Check sheet for the modelled part. Datum: model origin and axes. Units: mm. A direction names the side the tool comes from. Round coordinates to 2 decimals unless told otherwise and drop trailing zeros. Order: outer loops, then holes, each group sorted by start corner. A loop starts at its lowest first (then second) coordinate and runs counter-clockwise, first axis right, second up.
```python
from build123d import *

# Parameters (mm, degrees)
SKETCH3_R           = 2.225
BOSS_EXTRUDE1_DEPTH = 1.6


with BuildPart() as part:
    # Sketch1 → Revolve1 (revolve)
    with BuildSketch(Plane(origin=(0, 0, 0), x_dir=(1, 0, 0), z_dir=(0, 1, 0)), mode=Mode.PRIVATE) as revolve1_sk:
        with BuildLine():
            Line((0, -8.4), (0, 8.4))
            Line((0, 8.4), (1.725, 8.4))
            ThreePointArc((1.725, 8.4), (2.078553391, 8.253553391), (2.225, 7.9))
            Line((2.225, 7.9), (2.225, -7.9))
            ThreePointArc((2.225, -7.9), (2.078553391, -8.253553391), (1.725, -8.4))
            Line((1.725, -8.4), (0, -8.4))
        make_face()
    revolve(revolve1_sk.sketch.rotate(Axis((0, 0, -9.24), (0, 0, 1)), 180), axis=Axis((0, 0, -9.24), (0, 0, 1)))



with BuildPart() as body_2:
    # Sketch2 → Revolve2 (revolve)
    with BuildSketch(Plane.XZ, mode=Mode.PRIVATE) as revolve2_sk:
        with BuildLine():
            Line((-12.7, 8.4), (-14.425, 8.4))
            ThreePointArc((-14.425, 8.4), (-14.778553391, 8.253553391), (-14.925, 7.9))
            Line((-14.925, 7.9), (-14.925, -7.9))
            ThreePointArc((-14.925, -7.9), (-14.778553391, -8.253553391), (-14.425, -8.4))
            Line((-14.425, -8.4), (-12.7, -8.4))
            Line((-12.7, -8.4), (-12.7, 8.4))
        make_face()
    revolve(revolve2_sk.sketch.rotate(Axis((-12.7, 0, 8.4), (0, 0, -1)), 180), axis=Axis((-12.7, 0, 8.4), (0, 0, -1)))


with BuildPart() as part_1:
    add(part.part)

    add(body_2.part)  # Boss-Extrude1 merges body 2
    # Sketch3 → Boss-Extrude1 (add)
    with BuildSketch(Plane(origin=(0, 0, -5.475), x_dir=(0, -1, 0), z_dir=(0, 0, -1))):
        with BuildLine():
            ThreePointArc((-4.941202509, 2.635245294), (0, -5.6), (4.941202509, 2.635245294))
            ThreePointArc((4.941202509, 2.635245294), (4.012533333, 6.35), (4.941202509, 10.064754706))
            ThreePointArc((4.941202509, 10.064754706), (0, 18.3), (-4.941202509, 10.064754706))
            ThreePointArc((-4.941202509, 10.064754706), (-4.012533333, 6.35), (-4.941202509, 2.635245294))
        make_face()
        with Locations(Location((0, 0, 0), (0, 0, 90))):
            Circle(SKETCH3_R, mode=Mode.SUBTRACT)
        with Locations(Location((0, 12.7, 0), (0, 0, 270))):
            Circle(SKETCH3_R, mode=Mode.SUBTRACT)
    boss_extrude1 = extrude(amount=BOSS_EXTRUDE1_DEPTH)

    # Mirror1: Boss-Extrude1 across plane
    add(boss_extrude1.mirror(Plane.XY))


solid = part_1.part
```
Item 1: Access from +Z, -Z, +X, -X, +Y, -Y to the whole of each face (thin tool, end or side, straight path). Record for faces 1 (the flat face through (-7, 0, -5.475)), 2 (the cylindrical face through (-10.58, -0.67, 7.48)), 3 (the cylindrical face through (1.64, -1.504, -7.482)), 4 (the cylindrical face through (-6.404, 4.013, 6.264)), 5 (the cylindrical face through (-6.296, -4.013, 6.264)).
Answer:
face 1: none
face 2: +Z
face 3: -Z
face 4: +Z, -Z, +Y
face 5: +Z, -Z, -Y
Item 2: Sectioned sample at D-D (x = 0). Record the cut outline in (y, z) (3 decimals).
Answer:
outline: (-5.6, -7.075) - (-2.225, -7.075) - (-2.225, -7.9) arc R0.5 ccw to (-1.725, -8.4) - (1.725, -8.4) arc R0.5 ccw to (2.225, -7.9) - (2.225, -7.075) - (5.6, -7.075) - (5.6, -5.475) - (2.225, -5.475) - (2.225, 5.475) - (5.6, 5.475) - (5.6, 7.075) - (2.225, 7.075) - (2.225, 7.9) arc R0.5 ccw to (1.725, 8.4) - (-1.725, 8.4) arc R0.5 ccw to (-2.225, 7.9) - (-2.225, 7.075) - (-5.6, 7.075) - (-5.6, 5.475) - (-2.225, 5.475) - (-2.225, -5.475) - (-5.6, -5.475) - close
Item 3: Go/stop test with flat-tipped pins: P1, Ø1, axis at x = -3.5, z = -6.5, coming from the +Y side; P2, Ø6, axis at y = 0.5, z = 0, coming from the +X side (3 decimals); P3, Ø5, axis at x = -7.5, z = 5, coming from the +Y side. Record where each tip stops, or that it passes through.
Answer:
P1: stops at y = 4.76
P2: stops at x = 2.225
P3: stops at y = 4.88
Item 4: Release check for a two-part mould opening along Z. For faces 6 (the flat face through (-13, 0, -8.4)), 7 (the cylindrical face through (-10.58, -0.67, -0.08)), 8 (the flat face through (-7, 0, 7.075)), 9 (the cylindrical face through (-18.298, -0.162, -6.264)) record: released by +Z, released by -Z, zero draft, split by the parting line, or undercut.
Answer:
face 6: released by -Z
face 7: undercut
face 8: released by +Z
face 9: zero draft
Item 5: Scan lines: line 1 along Z through (x, y) = (-14.75, -4.25) (3 decimals); line 2 along X through (y, z) = (1.5, -4); line 3 along X through (y, z) = (2, -4) (3 decimals). Record each from-to range of solid material in increasing order.
Answer:
line 1: z = -7.075 to -5.475, 5.475 to 7.075
line 2: x = -14.34 to -11.06, -1.64 to 1.64
line 3: x = -13.675 to -11.725, -0.975 to 0.975
Item 6: Sectioned sample at C-C (z = 4.75). Record the cut outline in (x, y) (3 decimals).
Answer:
outline: circle Ø4.45 at (-12.7, 0); circle Ø4.45 at (0, 0)
Item 7: Sectioned sample at B-B (y = 3). Record the cut outline in (x, z) (3 decimals).
Answer:
outline: (-17.429, -7.075) - (4.729, -7.075) - (4.729, -5.475) - (-17.429, -5.475) - close; (-17.429, 5.475) - (4.729, 5.475) - (4.729, 7.075) - (-17.429, 7.075) - close
Item 8: Sectioned sample at A-A (x = -3.5). Record the cut outline in (y, z) (3 decimals).
Answer:
outline: (-4.545, -7.075) - (4.545, -7.075) - (4.545, -5.475) - (-4.545, -5.475) - close; (-4.545, 5.475) - (4.545, 5.475) - (4.545, 7.075) - (-4.545, 7.075) - close
